from build123d import *

# Parameters (mm, degrees)
BOSS_EXTRUDE1_DEPTH      = 5
BOSS_EXTRUDE1_DEPTH_BACK = 0.397201273
SKETCH1_W                = 70.9
SKETCH1_H                = 70.9
SKETCH1_R                = 5
SKETCH1_R_2              = 26
FILLET1_R                = 10


with BuildPart() as part:
    # Sketch1 → Boss-Extrude1 (new, two sides: drawn at the far end of the back side and taken through both)
    with BuildSketch(Plane.XY.offset(-BOSS_EXTRUDE1_DEPTH_BACK)):
        with Locations((35.45, 35.45)):
            Rectangle(SKETCH1_W, SKETCH1_H)
        with Locations((9.995, 60.905)):
            Circle(SKETCH1_R, mode=Mode.SUBTRACT)
        with Locations((60.905, 60.905)):
            Circle(SKETCH1_R, mode=Mode.SUBTRACT)
        with Locations((60.905, 9.995)):
            Circle(SKETCH1_R, mode=Mode.SUBTRACT)
        with Locations((9.995, 9.995)):
            Circle(SKETCH1_R, mode=Mode.SUBTRACT)
        with Locations((35.45, 35.45)):
            Circle(SKETCH1_R_2, mode=Mode.SUBTRACT)
    extrude(amount=BOSS_EXTRUDE1_DEPTH + BOSS_EXTRUDE1_DEPTH_BACK)

    # Fillet1
    fillet1_edges = [part.edges().sort_by_distance(p)[0] for p in [
        (0, 70.9, 2.301399364),
        (70.9, 70.9, 2.301399364),
        (70.9, 0, 2.301399364),
        (0, 0, 2.301399364),
    ]]
    fillet(fillet1_edges, radius=FILLET1_R)


solid = part.part
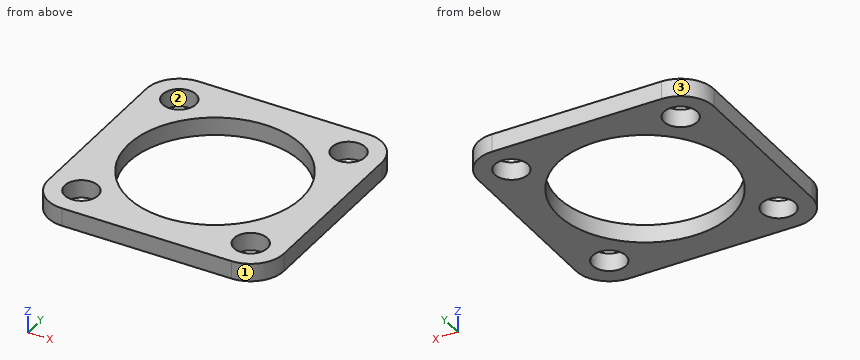
The listing builds one solid part. Answer for the finished solid, in the listing's coordinates (mm). Face numbers are marked on the shaded views. Give positions to 0.01 mm unless a question says otherwise; leave off trailing zeros. Order: outer loops, then holes, each group sorted by start corner. A loop starts at its lowest first (then second) coordinate and runs counter-clockwise, first axis right, second up. Notation, with made-up numbers: (74, 83) - (97, 83) arc R28 cw to (97, 113) - close; hole circle Ø3 at (64.5, 36). An arc over 180 degrees is marked (long way). One line per item, written item: value. Start each with the question number.
1) A cutting plane is placed at C-C on z = 1.25. Give the vertices of the cut face in (x, y) (3 decimals).
2) Given pin 1 Ø6 at (x, y) = (9.995, 60.905) entering from +Z, flat-ended and moving along its own axis, determine where the tip first touches the part or whether it passes through.
3) A cutting plane is placed at A-A on x = 35.45. Give the vertices of the cut face in (y, z), then the cut area to 3 significant figures.
4) The mould has two halves that part along Y. Classify the marked faces 1, 2 and 3: released by +Y, released by -Y, zero draft, split by the parting line, or undercut.
5) Find the intervals of material crossed by L1, parallel to X at y = 59.5, z = 1.25; L2, parallel to Y at x = 58, z = 3.6; L3, parallel to Y at x = 63, z = 0.45, in increasing order.
Answer sheet:
1. outline: (0, 10) arc R10 ccw to (10, 0) - (60.9, 0) arc R10 ccw to (70.9, 10) - (70.9, 60.9) arc R10 ccw to (60.9, 70.9) - (10, 70.9) arc R10 ccw to (0, 60.9) - close; hole circle Ø10 at (9.995, 9.995); hole circle Ø10 at (9.995, 60.905); hole circle Ø52 at (35.45, 35.45); hole circle Ø10 at (60.905, 9.995); hole circle Ø10 at (60.905, 60.905)
2. pin 1: passes through
3. outline: (0, -0.4) - (9.45, -0.4) - (9.45, 5) - (0, 5) - close; (61.45, -0.4) - (70.9, -0.4) - (70.9, 5) - (61.45, 5) - close
3. area: 102 mm2
4. face 1: released by -Y
4. face 2: undercut
4. face 3: released by +Y
5. L1: x = 0 to 5.2, 14.79 to 25.57, 45.33 to 56.11, 65.7 to 70.9
5. L2: y = 0 to 5.93, 14.06 to 22.51, 48.39 to 56.84, 64.97 to 70.9
5. L3: y = 0.22 to 5.46, 14.53 to 56.37, 65.44 to 70.68
